from build123d import *

# Parameters (mm, degrees)
BOSS_EXTRUDE1_DEPTH = 3
FILLET1_R           = 6
FILLET2_R           = 90
FILLET3_R           = 3
FILLET4_R           = 1
FILLET5_R           = 5
FILLET7_R           = 0.5


with BuildPart() as part:
    # Sketch1 → Boss-Extrude1 (new body)
    with BuildSketch(Plane(origin=(0, 0, 0), x_dir=(1, 0, 0), z_dir=(0, 1, 0))):
        with BuildLine():
            Line((26.26, 24.39), (21.003236337, 24.926095368))
            ThreePointArc((21.003236337, 24.926095368), (11.295062799, 23.773811444), (3, 18.6))
            Line((3, 18.6), (18.17, 16.74))
            Line((18.17, 16.74), (24.739702097, 17.401448676))
            ThreePointArc((24.739702097, 17.401448676), (26.605341282, 15.835769379), (24.991153908, 14.011938151))
            ThreePointArc((24.991153908, 14.011938151), (11.62395121, 11.060339085), (0, 3.83))
            Line((0, 3.83), (0, 0.53))
            ThreePointArc((0, 0.53), (9.076343052, 5.992821668), (19.42, 8.28))
            ThreePointArc((19.42, 8.28), (21.169232573, 6.746366569), (20.122543786, 4.668798598))
            Line((20.122543786, 4.668798598), (15.092493707, 2.268241119))
            ThreePointArc((15.092493707, 2.268241119), (14.296253692, 1.249322501), (14.63, 0))
            ThreePointArc((14.63, 0), (29.238150005, 2.169439215), (44, 2.607956962))
            ThreePointArc((44, 2.607956962), (47.61446857, 6.68515129), (49.32, 11.86))
            ThreePointArc((49.32, 11.86), (55.458987632, 13.234527387), (59.87, 17.72))
            ThreePointArc((59.87, 17.72), (54.010103044, 29.206202626), (41.4, 31.9))
            ThreePointArc((41.4, 31.9), (32.432757692, 30.961810725), (26.26, 24.39))
        make_face()
    extrude(amount=BOSS_EXTRUDE1_DEPTH)

    # Fillet1
    fillet1_edges = [part.edges().sort_by_distance(p)[0] for p in [
        (59.87, 1.5, -17.72),
    ]]
    fillet(fillet1_edges, radius=FILLET1_R)

    # Fillet2
    fillet2_edges = [part.edges().sort_by_distance(p)[0] for p in [
        (41.4, 1.5, -31.9),
    ]]
    fillet(fillet2_edges, radius=FILLET2_R)

    # Fillet3
    fillet3_edges = [part.edges().sort_by_distance(p)[0] for p in [
        (26.26, 1.5, -24.39),
        (0, 1.5, -3.83),
    ]]
    fillet(fillet3_edges, radius=FILLET3_R)

    # Fillet4
    fillet4_edges = [part.edges().sort_by_distance(p)[0] for p in [
        (49.32, 1.5, -11.86),
    ]]
    fillet(fillet4_edges, radius=FILLET4_R)

    # Fillet5
    fillet5_edges = [part.edges().sort_by_distance(p)[0] for p in [
        (44, 1.5, -2.607956962),
    ]]
    fillet(fillet5_edges, radius=FILLET5_R)

    # Fillet7
    fillet7_edges = [part.edges().sort_by_distance(p)[0] for p in [
        (14.63, 1.5, 0),
    ]]
    fillet(fillet7_edges, radius=FILLET7_R)


solid = part.part
CAD build for the part. Positions are in the model's coordinates, mm. A direction names the side the tool comes from. Give positions to 0.01 mm unless a question says otherwise; leave off trailing zeros. Order: outer loops, then holes, each group sorted by start corner. A loop starts at its lowest first (then second) coordinate and runs counter-clockwise, first axis right, second up. Notation, with made-up numbers: (78, 58.25) - (89, 58.25) arc R12 ccw to (89, 65.25) - close; hole circle Ø10 at (78.5, -4). An arc over 180 degrees is marked (long way). Write each question's results on one line, items separated by ' | '.
1. Probe L1, parallel to Z at x = 20.5, y = 1.3; L2, parallel to Z at x = 15, y = 0.95; L3, parallel to Z at x = 22.5, y = 2.35. List the from-to ranges inside material, lowest first. Write a range as from..to.
Calculated:
L1: z = -24.97..-16.97, -13.55..-7.86, -4.91..-1.08 | L2: z = -24.73..-17.13, -12.26..-7.73, -2.22..-0.08 | L3: z = -24.77..-17.18, -13.82..-1.39
2. Saw through at B-B on x = 54. List the corners of the cut face in (y, z), and give its area (3 significant figures).
Calculated:
outline: (0, -29.21) - (3, -29.21) - (3, -12.56) - (0, -12.56) - close | area: 50.0 mm2
3. Saw through at C-C on z = -29. List the corners of the cut face in (x, y), and give its area (3 significant figures).
Calculated:
outline: (29.54, 0) - (54.27, 0) - (54.27, 3) - (29.54, 3) - close | area: 74.2 mm2
4. Pull direction Z, two halves, no side cores. Call faces 1 (the face through (0.29, 1.52, -3.74)), 2 (the face through (12.46, 1.48, -11.39)), 3 (the face through (36, 0, -16)): released by +Z, released by -Z, zero draft, split by the parting line, or undercut.
Calculated:
face 1: released by -Z | face 2: undercut | face 3: zero draft
5. 3-axis set-ups, long thin cutter, end or side, ignore diameter. For faces 4 (the face through (22.63, 1.48, -24.76)), 5 (the face through (36, 3, -16)), 6 (the face through (10.479, 1.479, -17.683)), 7 (the face through (17.643, 1.479, -3.485)): which of +Z, -Z, +X, -X, +Y, -Y reach the whole face in a straight line?
Calculated:
face 4: -Z, +Y, -Y | face 5: +Z, -Z, +X, -X, +Y | face 6: -X, +Y, -Y | face 7: +Y, -Y
6. Pin check, flat tips, straight feed: pin 1 (1.5 mm diameter, centred on y = 1.5, z = -18.5, fed in from -X); pin 2 (1.5 mm diameter, centred on x = 6.5, y = 2.5, fed in from -Z). Stop position of each tip, or through.
Calculated:
pin 1: stops at x = 3 | pin 2: stops at z = -21.88
7. Saw through at A-A on z = -6. List the corners of the cut face in (x, y).
Calculated:
outline: (2.66, 0) - (9.09, 0) - (9.09, 3) - (2.66, 3) - close; (21.17, 0) - (47.19, 0) - (47.19, 3) - (21.17, 3) - close
